Check sheet for the modelled part. Datum: model origin and axes. Units: mm. A direction names the side the tool comes from. Round coordinates to 2 decimals unless told otherwise and drop trailing zeros. Order: outer loops, then holes, each group sorted by start corner. A loop starts at its lowest first (then second) coordinate and runs counter-clockwise, first axis right, second up. Notation, with made-up numbers: (19.5, 65.25) -> (40.5, 65.25) arc R22 ccw to (40.5, 71.25) -> close; hole circle Ø3 at (70, 12). An arc over 180 degrees is marked (long way). Answer in a Markdown table with one row per item. Add a question column.
1. Sectioned sample at B-B, the plane y = 19.05. Record the boundary of the cut face in (x, z), then the cut area to 3 significant figures.
2. Sectioned sample at C-C, the plane x = -17. Count the separate pieces of the cut face and the enclosed holes in it, then the cut area to 3 significant figures.
3. Material ranges on L1, parallel to Z at x = -7, y = 19.05; L2, parallel to Z at x = -25.5, y = 19.05; L3, parallel to Y at x = -40, z = -63.5 (3 decimals), recorded low to high. Write a range as from..to.
4. Depth check by flat-ended pin: P1, Ø6, axis at y = 19.05, z = 63.5, coming from the +X side; P2, Ø11.5, axis at y = 136.525, z = -63.5, coming from the -X side; P3, Ø3, axis at x = -30.5, z = -39.5, coming from the -Y side (3 decimals). Enter the tip coordinate at first touch or a pass-through.
5. Access from +Z, -Z, +X, -X, +Y, -Y to the whole of each face (thin tool, end or side, straight path). Record for faces 1 (the flat face through (-24, 0, 57.15)), 2 (the flat face through (0, 36.8, 62.4)), 3 (the cylindrical face through (-25.11, 131.82, 58.97)), 4 (the flat face through (-8.89, 21, 61)).
6. Draft check along Z on faces 5 (the flat face through (-24, 14, -69.85)), 6 (the flat face through (-46.399, -101.556, 65.987)), 7 (the cylindrical face through (-24.418, 141.064, 67.94)), 8 (the cylindrical face through (-4.507, 18.827, 68.575)). Enter one of: +Z half, -Z half, draft (parallel to the pull), parting line (faces both ways), or undercut.
7. Sectioned sample at A-A, the plane y = -43.5. Record the boundary of the cut face in (x, z).
8. Sectioned sample at D-D, the plane z = -47. Record the boundary of the cut face in (x, y) (3 decimals).
Autodesk Inventor part; units mm, degrees
ref_plane "YZ Plane" through (0, 0, 0) normal (1, 0, 0) x (0, 1, 0)
ref_plane "XZ Plane" through (0, 0, 0) normal (0, 1, 0) x (-1, 0, 0)
ref_plane "XY Plane" through (0, 0, 0) normal (0, 0, 1) x (1, 0, 0)
sketch "Sketch1" plane through (0, 0, 0) normal (1, 0, 0) x (0, 1, 0)
  line L0 (0, 99.6312) -> (0, -99.6312)
  line L1 (-202.2597, 0) -> (204.2274, 0)
  line L2 (-136.525, -69.85) -> (136.525, -69.85)
  line L3 (142.875, -63.5) -> (142.875, 63.5)
  line L4 (136.525, 69.85) -> (-136.525, 69.85)
  line L5 (-142.875, 63.5) -> (-142.875, -63.5)
  line L6 (-142.875, -69.85) -> (142.875, 69.85) construction
  line L7 (142.875, -69.85) -> (-142.875, 69.85) construction
  arc A0 (142.875, 63.5) -> (136.525, 69.85) centre (136.525, 63.5) ccw
  arc A1 (136.525, -69.85) -> (142.875, -63.5) centre (136.525, -63.5) ccw
  arc A2 (-142.875, -63.5) -> (-136.525, -69.85) centre (-136.525, -63.5) ccw
  arc A3 (-136.525, 69.85) -> (-142.875, 63.5) centre (-136.525, 63.5) ccw
  line L8 (130.175, 57.15) -> (130.175, -57.15)
  line L9 (130.175, -57.15) -> (-130.175, -57.15)
  line L10 (-130.175, -57.15) -> (-130.175, 57.15)
  line L11 (-130.175, 57.15) -> (130.175, 57.15)
  line L12 (-136.525, 63.5) -> (136.525, 63.5) construction
  line L13 (136.525, 63.5) -> (136.525, -63.5) construction
  line L14 (136.525, -63.5) -> (-136.525, -63.5) construction
  line L15 (-136.525, -63.5) -> (-136.525, 63.5) construction
  line L16 (-136.525, 63.5) -> (136.525, -63.5) construction
  line L17 (136.525, 63.5) -> (-136.525, -63.5) construction
  point P0 (0, 0)
  point P1 (19.05, 63.5)
  point P2 (19.05, -63.5)
  point P3 (-19.05, 63.5)
  point P4 (-19.05, -63.5)
  dimension "d0" = 139.7
  dimension "d1" = 285.75
  dimension "d2" = 6.35
  dimension "d3" = 12.7
  dimension "d4" = 6.35
  dimension "d5" = 6.35
  dimension "d6" = 19.05
  dimension "d7" = 19.05
extrude "Extrusion1" add sketch "Sketch1" against normal blind 49.53 contours L4 A0 L3 L1 L8 L11 L0 | L0 L11 L10 L1 L5 A3 L4 | L9 L8 L1 L3 A1 L2 L0 | L0 L2 A2 L5 L1 L10 L9
fillet "Fillet1" radius 6.35 4 edges at (-24.765, 130.175, 57.15) (-24.765, 130.175, -57.15) (-24.765, -130.175, -57.15) (-24.765, -130.175, 57.15)
hole "Hole1" at (0, 136.525, 63.5) at (0, 136.525, -63.5) at (0, 19.05, 63.5) at (0, 19.05, -63.5) at (0, -19.05, 63.5) at (0, -19.05, -63.5) at (0, -136.525, 63.5) at (0, -136.525, -63.5) direction (-1, 0, 0) diameter 5.334 end through all counterbore diameter 10.16 counterbore depth 8.89
sketch "Sketch2" plane through (-49.53, 0, 0) normal (-1, 0, 0) x (0, 0, 1)
  line L0 (0, -202.2597) -> (0, 204.2274)
  line L1 (99.6312, 0) -> (-99.6312, 0)
  line L2 (119.4093, -203.1024) -> (-119.4093, -203.1024)
  line L3 (-119.4093, -203.1024) -> (-119.4093, 0)
  line L4 (-119.4093, 0) -> (119.4093, 0)
  line L5 (119.4093, 0) -> (119.4093, -203.1024)
  line L6 (119.4093, -203.1024) -> (-119.4093, 0) construction
  line L7 (-119.4093, -203.1024) -> (119.4093, 0) construction
  point P0 (0, 0)
  point P1 (0, -101.5512)
  point P2 (119.4093, 0)
  dimension "d18" = 0
extrude "Extrusion2" [suppressed]
sketch "Sketch3" plane through (-34.925, 0, -69.85) normal (0, -1, 0) x (1, 0, 0)
  line L0 (0, 12.7) -> (34.925, 12.7)
  line L1 (0, 0) -> (0, 12.7)
  line L2 (34.925, 0) -> (0, 0)
  line L3 (34.925, 12.7) -> (34.925, 0)
  line L4 (34.925, 127) -> (0, 127)
  line L5 (34.925, 139.7) -> (34.925, 127)
  line L6 (0, 139.7) -> (34.925, 139.7)
  line L7 (0, 127) -> (0, 139.7)
  line L8 (0, 133.35) -> (0, 6.35) construction
  line L9 (34.925, 6.35) -> (0, 6.35) construction
  line L10 (0, 6.35) -> (34.925, 6.35) construction
  line L11 (0, 133.35) -> (34.925, 133.35) construction
  line L12 (34.925, 135.417) -> (34.925, 131.283) construction
  line L13 (34.925, 133.35) -> (0, 133.35) construction
  point P0 (34.925, 69.85)
  point P1 (7.62, 6.35)
  point P2 (27.305, 6.35)
  point P3 (27.305, 133.35)
  point P4 (7.62, 133.35)
  dimension "d21" = 7.62
  dimension "d22" = 7.62
  dimension "d23" = 7.62
  dimension "d24" = 7.62
hole "Hole2" [suppressed]
chamfer "Chamfer1" [suppressed]
sketch "Sketch4" plane through (-49.53, 0, 0) normal (-1, 0, 0) x (0, 0, 1)
  line L0 (0, -202.2597) -> (0, 204.2274)
  line L1 (99.6312, 0) -> (-99.6312, 0)
  line L2 (116.354, -104.775) -> (-116.354, -104.775)
  line L3 (-116.354, -104.775) -> (-116.354, -199.2224)
  line L4 (-116.354, -199.2224) -> (116.354, -199.2224)
  line L5 (116.354, -199.2224) -> (116.354, -104.775)
  line L6 (116.354, -104.775) -> (-116.354, -199.2224) construction
  line L7 (-116.354, -104.775) -> (116.354, -199.2224) construction
  line L8 (63.5, 142.875) -> (-63.5, 142.875)
  point P0 (0, 0)
  point P1 (0, -151.9987)
  dimension "d35" = 247.65
extrude "Extrusion3" cut sketch "Sketch4" against normal through all
sketch "Sketch5" plane through (-49.53, 0, 0) normal (-1, 0, 0) x (0, 0, 1)
  line L0 (-57.15, -104.775) -> (-57.15, 123.825)
  line L1 (-50.8, 130.175) -> (50.8, 130.175)
  line L2 (57.15, 123.825) -> (57.15, -104.775)
  line L3 (0, -202.2597) -> (0, 204.2274)
  arc A0 (-50.8, 130.175) -> (-57.15, 123.825) centre (-50.8, 123.825) ccw
  arc A1 (57.15, 123.825) -> (50.8, 130.175) centre (50.8, 123.825) ccw
  line L4 (-62.23, -104.775) -> (-62.23, 123.825)
  arc A2 (-50.8, 135.255) -> (-62.23, 123.825) centre (-50.8, 123.825) ccw
  line L5 (-50.8, 135.255) -> (50.8, 135.255)
  arc A3 (62.23, 123.825) -> (50.8, 135.255) centre (50.8, 123.825) ccw
  line L6 (62.23, 123.825) -> (62.23, -104.775)
  line L7 (62.23, -28.575) -> (-62.23, -28.575)
  line L8 (-62.23, -28.575) -> (-62.23, 28.575)
  line L9 (-62.23, 28.575) -> (62.23, 28.575)
  line L10 (62.23, 28.575) -> (62.23, -28.575)
  line L11 (62.23, -28.575) -> (-62.23, 28.575) construction
  line L12 (-62.23, -28.575) -> (62.23, 28.575) construction
  line L13 (-69.85, -104.775) -> (-57.15, -104.775)
  line L14 (57.15, -104.775) -> (69.85, -104.775)
  point P0 (0, 0)
  point P1 (57.15, 28.575)
  point P2 (-57.15, 28.575)
  point P3 (57.15, -28.575)
  point P4 (-57.15, -28.575)
  dimension "d38" = 5.08
  dimension "d39" = 57.15
extrude "Extrusion4" cut sketch "Sketch5" against normal through all contours L13 L4 L7 L0 | L9 L4 A2 L5 L3 L1 A0 L0 | L7 L6 L14 L2 | L3 L5 A3 L6 L9 L2 A1 L1
fillet "Fillet2" radius 3.175 8 edges at (-24.765, -28.575, -57.15) (-24.765, -28.575, -62.23) (-24.765, 28.575, -57.15) (-24.765, 28.575, -62.23) (-24.765, -28.575, 57.15) (-24.765, -28.575, 62.23) (-24.765, 28.575, 57.15) (-24.765, 28.575, 62.23)
chamfer "Chamfer2" distance 6.35 angle 45 2 edges at (-49.53, -104.775, -66.04) (-49.53, -104.775, 66.04)
sketch "Sketch6" plane through (-49.53, 0, 0) normal (-1, 0, 0) x (0, 0, 1)
  line L0 (69.0599, 146.1578) -> (-63.5, 146.1578) construction
  line L1 (-63.5, 146.1578) -> (-63.5, -84.3884) construction
  line L2 (-63.5, -84.3884) -> (69.0599, -84.3884) construction
  line L3 (69.0599, -84.3884) -> (69.0599, 146.1578) construction
  line L4 (69.0599, 146.1578) -> (-63.5, -84.3884) construction
  line L5 (-63.5, 146.1578) -> (69.0599, -84.3884) construction
  point P0 (0, 0)
  point P1 (2.7799, 30.8847)
  point P2 (63.5, -19.05)
  point P3 (-63.5, 136.525)
Answer key:
| question | item | result |
|---|---|---|
| 1 | outline | (-49.53, -69.85) -> (0, -69.85) -> (0, -68.58) -> (-8.89, -68.58) -> (-8.89, -66.17) -> (-49.53, -66.17) -> close; (-49.53, -60.83) -> (-8.89, -60.83) -> (-8.89, -58.42) -> (0, -58.42) -> (0, -57.15) -> (-49.53, -57.15) -> close; (-49.53, 57.15) -> (0, 57.15) -> (0, 58.42) -> (-8.89, 58.42) -> (-8.89, 60.83) -> (-49.53, 60.83) -> close; (-49.53, 66.17) -> (-8.89, 66.17) -> (-8.89, 68.58) -> (0, 68.58) -> (0, 69.85) -> (-49.53, 69.85) -> close |
| 1 | area | 644 mm² |
| 2 | separate pieces | 1 |
| 2 | enclosed holes | 6 |
| 2 | area | 5,210 mm² |
| 3 | L1 | z = -69.85..-68.58, -58.42..-57.15, 57.15..58.42, 68.58..69.85 |
| 3 | L2 | z = -69.85..-66.17, -60.83..-57.15, 57.15..60.83, 66.17..69.85 |
| 3 | L3 | y = -104.775..-21.717, -16.383..16.383, 21.717..133.858, 139.192..142.875 |
| 4 | P1 | stops at x = -8.89 |
| 4 | P2 | stops at x = -49.53 |
| 4 | P3 | stops at y = 135.255 |
| 5 | face 1 | +X, -X, -Y |
| 5 | face 2 | +Z, -Z, +X, +Y, -Y |
| 5 | face 3 | +X, -X |
| 5 | face 4 | +X |
| 6 | face 5 | -Z half |
| 6 | face 6 | draft |
| 6 | face 7 | +Z half |
| 6 | face 8 | undercut |
| 7 | outline | (-49.53, -69.85) -> (0, -69.85) -> (0, -62.23) -> (-49.53, -62.23) -> close; (-49.53, 62.23) -> (0, 62.23) -> (0, 69.85) -> (-49.53, 69.85) -> close |
| 8 | outline | (-49.53, 135.255) -> (0, 135.255) -> (0, 142.875) -> (-49.53, 142.875) -> close |
